from build123d import *

# Parameters (mm, degrees)
F0_W     = 129
F0_H     = 15
F1_DEPTH = 170
F3_D     = 6
F5_D     = 4.2
F5_DEPTH = 15
F5_TIP   = 1.2618073
F6_DEPTH = 5
F7_DEPTH = 5
F8_DEPTH = 5


with BuildPart() as f1:
    # F0 (on Right) → F1 (new body)
    with BuildSketch(Plane.YZ):
        with Locations((64.5, 7.5)):
            Rectangle(F0_W, F0_H)
    extrude(amount=F1_DEPTH)

    # F3 (through all)
    with Locations(Plane(origin=(0, 0, 0), x_dir=(1, 0, 0), z_dir=(0, 0, -1))):
        with Locations((13, -6), (13, -38), (49, -6), (49, -38), (121, -38), (121, -6), (157, -6), (157, -38)):
            Hole(F3_D / 2)

    # F5
    with Locations(Plane(origin=(0, 129, 0), x_dir=(-1, 0, 0), z_dir=(0, 1, 0))):
        with Locations((-151, 7.5), (-85, 7.5), (-118, 7.5), (-52, 7.5), (-19, 7.5)):
            Hole(F5_D / 2, depth=F5_DEPTH)
            with Locations((0, 0, -(F5_DEPTH + F5_TIP / 2))):  # 118° drill point
                Cone(0, F5_D / 2, F5_TIP, mode=Mode.SUBTRACT)

    # F6 (add): a face of the model
    f6_faces = [f1.faces().sort_by_distance(p)[0] for p in [
        (170, 64.5, 7.5),
    ]]
    extrude(f6_faces, amount=F6_DEPTH)

    # F7 (add): a face of the model
    f7_faces = [f1.faces().sort_by_distance(p)[0] for p in [
        (0, 64.5, 7.5),
    ]]
    extrude(f7_faces, amount=F7_DEPTH)

    # F8 (add): a face of the model
    f8_faces = [f1.faces().sort_by_distance(p)[0] for p in [
        (85, 0, 7.5),
    ]]
    extrude(f8_faces, amount=F8_DEPTH)


solid = f1.part
Can you work these out from the model? Positions are in its coordinate system, mm. A direction names the side the tool comes from. Give positions to 0.01 mm unless a question says otherwise; leave off trailing zeros. Write each loop counter-clockwise with the first axis right and the second up, starting at its lowest first coordinate (ties: lowest second). Pieces come first, ordered by that corner, then holes. Notation, with made-up numbers: (9.25, 88) -> (62.25, 88) arc R10 cw to (62.25, 100) -> close; hole circle Ø8 at (37.5, -7). An arc over 180 degrees is marked (long way). Answer as a JSON object with one key per item and string values. Group by question number.
Item 1: I'm going to push flat-ended pins straight in: P1, Ø2.5, axis at x = 118, z = 7.5, coming from the +Y side; P2, Ø3.5, axis at x = 151, z = 7.5, coming from the +Y side. Where does each tip first touch, or does it pass through?
Item 2: Suppose I cut it at A-A (y = 6). Please give me the cut outline in (x, z).
Item 3: Please list where these lines run through material, in increasing order: line 1 (X direction, y = 123.25, z = 7.5); line 2 (Y direction, x = 49, z = 3.25); line 3 (X direction, y = 38, z = 8). Write a range as [from, to].
Item 4: We'd pull the mould along Y, two halves only. Please class faces 1 (the face through (154.14, 37.1, 7.6)), 2 (the face through (84, 63, 0)), 3 (the face through (86, 129, 4)): +Y half, -Y half, draft (parallel to the pull), parting line (faces both ways), or undercut.
Item 5: For faces 4 (the face through (-5, 63, 7)), 5 (the face through (21.003, 121.395, 8.131)), which set-ups out of +Z, -Z, +X, -X, +Y, -Y let a thin tool reach every point of the face, with its end or its side?
Findings:
{
 "1": {"P1": "stops at y = 113.49", "P2": "stops at y = 113.79"},
 "2": {"outline": "(-5, 0) -> (10, 0) -> (10, 15) -> (-5, 15) -> close; (16, 0) -> (46, 0) -> (46, 15) -> (16, 15) -> close; (52, 0) -> (118, 0) -> (118, 15) -> (52, 15) -> close; (124, 0) -> (154, 0) -> (154, 15) -> (124, 15) -> close; (160, 0) -> (175, 0) -> (175, 15) -> (160, 15) -> close"},
 "3": {"line 1": "x = [-5, 16.9], [21.1, 49.9], [54.1, 82.9], [87.1, 115.9], [120.1, 148.9], [153.1, 175]", "line 2": "y = [-5, 3], [9, 35], [41, 129]", "line 3": "x = [-5, 10], [16, 46], [52, 118], [124, 154], [160, 175]"},
 "4": {"face 1": "undercut", "face 2": "draft", "face 3": "+Y half"},
 "5": {"face 4": "+Z, -Z, -X, +Y, -Y", "face 5": "+Y"}
}
